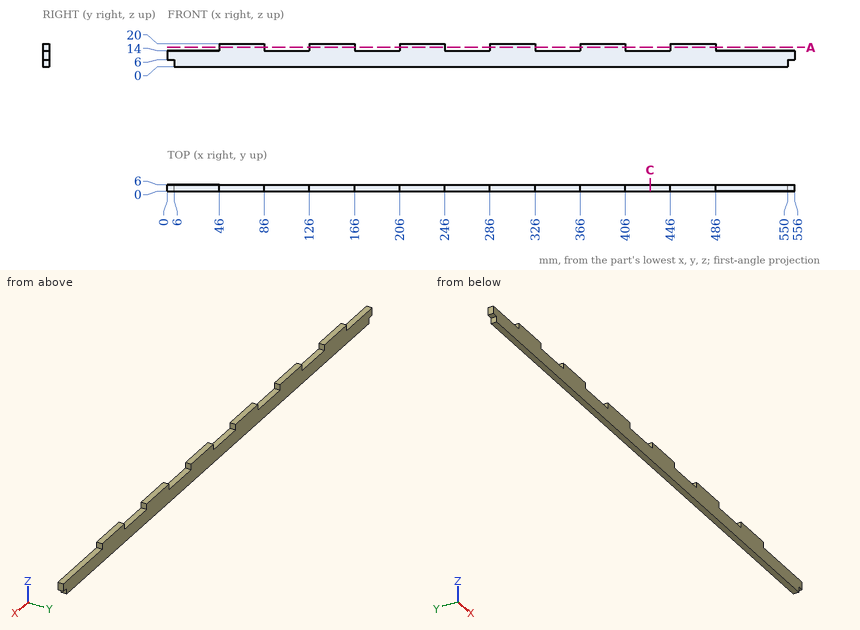
Job drawing, mm, ordinate dimensions from the low corner. One solid piece. Give positions to 0.01 mm unless a question says otherwise; leave off trailing zeros. Loops run counter-clockwise (first coordinate to the right, second up) from the corner with the lowest first, then second, coordinate; pieces in that order, holes last.
Item 1: Slice it at A-A, the plane z = 17. List the corners of the cut face in (x, y), and give its area (3 significant figures).
Answers follow:
outline: (46, 0) - (86, 0) - (86, 6) - (46, 6) - close; (126, 0) - (166, 0) - (166, 6) - (126, 6) - close; (206, 0) - (246, 0) - (246, 6) - (206, 6) - close; (286, 0) - (326, 0) - (326, 6) - (286, 6) - close; (366, 0) - (406, 0) - (406, 6) - (366, 6) - close; (446, 0) - (486, 0) - (486, 6) - (446, 6) - close
area: 1,440 mm2
Item 2: Slice it at C-C, the plane x = 428. List the corners of the cut face in (y, z), and give its area (3 significant figures).
Answers follow:
outline: (0, 0) - (6, 0) - (6, 14) - (0, 14) - close
area: 84.0 mm2
Item 3: Flat gauge pins, fed straight in: pin 1 (1.8 mm diameter, centred on y = 3.5, z = 15.5, fed in from +X); pin 2 (3 mm diameter, centred on x = 351.5, y = 3.5, fed in from +Z); pin 3 (4 mm diameter, centred on x = 486.5, z = 2, fed in from -Y); pin 4 (1.8 mm diameter, centred on y = 1.5, z = 16.5, fed in from -X). Where does each tip first touch, or does it go through?
Answers follow:
pin 1: stops at x = 486
pin 2: stops at z = 14
pin 3: stops at y = 0
pin 4: stops at x = 46
Item 4: Drill centre lines: line 1 (X direction, y = 2.2, z = 18.5); line 2 (Z direction, x = 23, y = 4); line 3 (X direction, y = 4.05, z = 4). Where is each one in solid material? Low to high.
Answers follow:
line 1: x = 46 to 86, 126 to 166, 206 to 246, 286 to 326, 366 to 406, 446 to 486
line 2: z = 0 to 14
line 3: x = 6 to 550
